CAD build for the part. Positions are in the model's coordinates, mm. Coordinates: 2 decimals unless noted, no trailing zeros. Order: outer loops, then holes, each group sorted by start corner. A loop starts at its lowest first (then second) coordinate and runs counter-clockwise, first axis right, second up. Notation, with made-up numbers: M -1.75,39 L 26.25,39 A21 ccw 26.25,54 Z; hole C 55,0 d3. An arc over 180 degrees is marked long. One line per item, written item: value.
from build123d import *

# Parameters (mm, degrees)
F1_DEPTH = 25.4
F2_R     = 12.69999


# Not quite as in the source:
# - a fillet or chamfer is up to 0.001 mm smaller than in the source, because OpenCascade refuses the exact size


with BuildPart() as f1:
    # F0 (on Top) → F1 (new body)
    with BuildSketch(Plane.XY):
        Polygon((51.9719609901, 29.8469270905), (0.1377834097, 59.9325020472), (-51.8341775803, 30.0855749566), (-51.9719609901, -29.8469270905), (-0.1377834097, -59.9325020472), (51.8341775803, -30.0855749566), align=None)
    extrude(amount=F1_DEPTH)

    # F2 (radius 12.7 in the source; OpenCascade refuses exactly that, so slightly less here)
    f2_edges = [f1.edges().sort_by_distance(p)[0] for p in [
        (51.971961, 29.846927, 12.7),
        (0.137783, 59.932502, 12.7),
        (26.054872, 44.889715, 0),
        (26.054872, 44.889715, 25.4),
        (-51.834178, 30.085575, 12.7),
        (-25.848197, 45.009039, 0),
        (-25.848197, 45.009039, 25.4),
        (-51.971961, -29.846927, 12.7),
        (-51.903069, 0.119324, 0),
        (-51.903069, 0.119324, 25.4),
        (-0.137783, -59.932502, 12.7),
        (51.834178, -30.085575, 12.7),
        (25.848197, -45.009039, 0),
        (25.848197, -45.009039, 25.4),
        (-26.054872, -44.889715, 0),
        (-26.054872, -44.889715, 25.4),
        (51.903069, -0.119324, 0),
        (51.903069, -0.119324, 25.4),
    ]]
    fillet(f2_edges, radius=F2_R)


solid = f1.part
Q1. Slice it at A-A (z = 2.25). List the corners of the cut face in (x, y).
Recorded:
outline: M -46.47,-22.53 A7.22 ccw -42.88,-28.79 L -3.73,-51.51 A7.22 ccw 3.49,-51.53 L 42.75,-28.98 A7.22 ccw 46.37,-22.74 L 46.47,22.53 A7.22 ccw 42.88,28.79 L 3.73,51.51 A7.22 ccw -3.49,51.53 L -42.75,28.98 A7.22 ccw -46.37,22.74 Z
Q2. Drill centre lines: line 1 along Y through (x, z) = (-34, 6.25); line 2 along X through (y, z) = (-40.5, 17.5); line 3 along Y through (x, z) = (-7, 23). Where is each one in solid material? Low to high.
Recorded:
line 1: y = -38.24 to 38.3
line 2: x = -31.74 to 31.81
line 3: y = -49.86 to 49.76
Q3. Slice it at B-B (z = 22.5). List the corners of the cut face in (x, y), plus the area to 3 significant figures.
Recorded:
outline: M -47.33,-22.53 A8.08 ccw -43.31,-29.53 L -4.16,-52.25 A8.08 ccw 3.92,-52.27 L 43.17,-29.73 A8.08 ccw 47.23,-22.74 L 47.33,22.53 A8.08 ccw 43.31,29.53 L 4.16,52.25 A8.08 ccw -3.92,52.27 L -43.17,29.73 A8.08 ccw -47.23,22.74 Z
area: 7,720 mm^2
Q4. Pin check, flat tips, straight feed: pin 1 Ø4 at (x, y) = (-34.5, -29) entering from -Z; pin 2 Ø8 at (y, z) = (-26.5, 23) entering from +X; pin 3 Ø3 at (y, z) = (28.5, 2.5) entering from +X; pin 4 Ø1 at (x, y) = (24, 28.5) entering from -Z. Stop position of each tip, or through.
Recorded:
pin 1: stops at z = 0.06
pin 2: stops at x = 49.77
pin 3: stops at x = 46.67
pin 4: stops at z = 0
